Autodesk Inventor part; units mm, degrees
ref_plane "YZ Plane" through (0, 0, 0) normal (1, 0, 0) x (0, 1, 0)
ref_plane "XZ Plane" through (0, 0, 0) normal (0, 1, 0) x (-1, 0, 0)
ref_plane "XY Plane" through (0, 0, 0) normal (0, 0, 1) x (1, 0, 0)
sketch "Sketch1" plane through (0, 0, 0) normal (0, 0, 1) x (1, 0, 0)
  line L0 (-17.78, 0) -> (17.78, 0)
  line L1 (0, -17.78) -> (0, 17.78)
  line L2 (-12.7, 12.7) -> (12.7, 12.7)
  line L3 (12.7, 12.7) -> (12.7, -12.7)
  line L4 (12.7, -12.7) -> (-12.7, -12.7)
  line L5 (-12.7, -12.7) -> (-12.7, 12.7)
  line L6 (9.525, 9.525) -> (-9.525, 9.525)
  line L7 (-9.525, 9.525) -> (-9.525, -9.525)
  line L8 (-9.525, -9.525) -> (9.525, -9.525)
  line L9 (9.525, -9.525) -> (9.525, 9.525)
  point P0 (0, 0)
  point P1 (-12.7, 0)
  point P2 (0, 12.7)
  dimension "d0" = 25.4
  dimension "d1" = 3.175
extrude "Extrusion1" add sketch "Sketch1" along normal mid plane 279.4 contours L5 L2 L1 L6 L7 L0 | L0 L7 L8 L1 L4 L5 | L1 L8 L9 L0 L3 L4 | L2 L3 L0 L9 L6 L1
sketch "Sketch3" plane through (-12.7, 12.7, 139.7) normal (0, 1, 0) x (1, 0, 0)
  line L0 (0, 0) -> (25.4, 0)
  line L1 (25.4, 0) -> (25.4, 279.4)
  line L2 (0, 0) -> (25.4, 14.6647)
  point P0 (12.7, 139.7)
  dimension "d7" = 30
extrude "Extrusion3" cut sketch "Sketch3" against normal through all
sketch "Sketch4" plane through (-12.7, 12.7, -139.7) normal (0, 1, 0) x (1, 0, 0)
  line L0 (25.4, -264.7353) -> (25.4, 0)
  line L1 (25.4, 0) -> (0, 0)
  line L2 (0, 0) -> (25.4, -43.9941)
  point P0 (12.7, -139.7)
  dimension "d10" = 60
extrude "Extrusion4" cut sketch "Sketch4" against normal through all
properties part number "tubing_template_0.125" material "Aluminum-6061"
Here's how the part is built. I have some questions about the finished solid (model axes, mm). A direction names the side the tool comes from. Coordinates: 2 decimals unless noted, no trailing zeros. Order: outer loops, then holes, each group sorted by start corner. A loop starts at its lowest first (then second) coordinate and runs counter-clockwise, first axis right, second up.
Item 1: For faces 1 (the face through (0, -9.525, 0)), 2 (the face through (0, -12.7, -2)), which set-ups out of +Z, -Z, +X, -X, +Y, -Y let a thin tool reach every point of the face, with its end or its side?
Result sheet:
face 1: +Z, -Z
face 2: +Z, -Z, +X, -X, -Y
Item 2: If we section it at C-C on x = -7: List the corners of the cut face in (y, z) for me (3 decimals).
Result sheet:
outline: (-12.7, -129.827) - (-9.525, -129.827) - (-9.525, 136.409) - (-12.7, 136.409) - close; (9.525, -129.827) - (12.7, -129.827) - (12.7, 136.409) - (9.525, 136.409) - close
Item 3: If we section it at A-A on y = -5.25: List the corners of the cut face in (x, z) for me (3 decimals).
Result sheet:
outline: (-12.7, -139.7) - (-9.525, -134.201) - (-9.525, 137.867) - (-12.7, 139.7) - close; (9.525, -101.205) - (12.7, -95.706) - (12.7, 125.035) - (9.525, 126.868) - close
Item 4: For P1, Ø5, axis at x = -7.5, y = -3.5, coming from the -Z side; P2, Ø3, axis at x = -3.5, y = -9, coming from the +Z side, each with a flat end and sliding along its axis, tell me the tip position at first contact or that it passes through.
Result sheet:
P1: stops at z = -135.02
P2: stops at z = 135.2
Item 5: If we mould it in two halves opening along Y, with no side actions, what happens to faces 3 (the face through (9.525, 0, 11)), 4 (the face through (0, 12.7, -2)), 5 (the face through (-0.178, -11.111, -118.011))? For each: +Y half, -Y half, draft (parallel to the pull), parting line (faces both ways), or undercut.
Result sheet:
face 3: undercut
face 4: +Y half
face 5: draft
Item 6: I need wall thicknesses on line 1 (Y direction, x = 0.75, z = -102) (3 decimals); line 2 (X direction, y = 6, z = -108) (3 decimals). Which ranges of each line are inside material? Lowest first, please.
Result sheet:
line 1: y = -12.7 to -9.525, 9.525 to 12.7
line 2: x = -12.7 to -9.525
Item 7: If we section it at B-B on z = 23: List the corners of the cut face in (x, y) for me (3 decimals).
Result sheet:
outline: (-12.7, -12.7) - (12.7, -12.7) - (12.7, 12.7) - (-12.7, 12.7) - close; hole (-9.525, -9.525) - (9.525, -9.525) - (9.525, 9.525) - (-9.525, 9.525) - close
